Source: CAD feature listing. Evaluate the final solid. Frame: model axes, mm. Round coordinates to 2 decimals unless told otherwise and drop trailing zeros. Loops run counter-clockwise (first coordinate to the right, second up) from the corner with the lowest first, then second, coordinate; pieces in that order, holes last.
Item 1: Ray query, L1, parallel to Z at x = 95, y = 1.05; L2, parallel to X at y = 1.25, z = 52; L3, parallel to X at y = 4.15, z = -26 (3 decimals). Return the intervals inside material, ascending.
Item 2: Section query C-C on x = -34.5. Return loops of the section in (y, z).
Item 3: First-contact query: P1, Ø2.5, axis at x = -94.5, z = -52, coming from the +Y side; P2, Ø1.6, axis at y = 4, z = 14, coming from the +X side; P3, Ø0.6, axis at x = 50, y = 4.5, coming from the -Z side. Flat tips, straight axial feed; report the tip coordinate or a pass-through.
Item 4: Section query D-D on x = -80. Return loops of the section in (y, z).
Item 5: Section query B-B on y = 3.8. Return loops of the section in (x, z) (3 decimals), then the cut area to 3 significant figures.
Item 6: Section query A-A on z = -26. Return loops of the section in (x, y) (3 decimals).
```python
from build123d import *

# Parameters (mm, degrees)
SKETCH1_W           = 195
SKETCH1_H           = 110
BOSS_EXTRUDE1_DEPTH = 3
BOSS_EXTRUDE2_DEPTH = 2
SKETCH4_R           = 1.5
CUT_EXTRUDE2_DEPTH  = 112.983257677
FILLET1_R           = 3
SKETCH5_R           = 1.5
CUT_EXTRUDE3_DEPTH  = 113.054674155
SKETCH6_R           = 10.35
CUT_EXTRUDE4_DEPTH  = 113.054674155
SKETCH7_R           = 11.4
CUT_EXTRUDE5_DEPTH  = 2


with BuildPart() as part:
    # Sketch1 → Boss-Extrude1 (new body)
    with BuildSketch(Plane(origin=(0, 0, 0), x_dir=(1, 0, 0), z_dir=(0, 1, 0))):
        Rectangle(SKETCH1_W, SKETCH1_H)
    extrude(amount=BOSS_EXTRUDE1_DEPTH)

    # Sketch2 → Boss-Extrude2 (add)
    with BuildSketch(Plane(origin=(0, 3, 0), x_dir=(1, 0, 0), z_dir=(0, 1, 0))):
        with BuildLine():
            Line((-94.5, 0), (-94.5, 49))
            ThreePointArc((-94.5, 49), (-92.378679656, 49.878679656), (-91.5, 52))
            Line((-91.5, 52), (-13, 52))
            ThreePointArc((-13, 52), (-10.878679656, 51.121320344), (-10, 49))
            Line((-10, 49), (-10, -49))
            ThreePointArc((-10, -49), (-10.878679656, -51.121320344), (-13, -52))
            Line((-13, -52), (-91.5, -52))
            ThreePointArc((-91.5, -52), (-92.378679656, -49.878679656), (-94.5, -49))
            Line((-94.5, -49), (-94.5, 0))
        make_face()
        with BuildLine():
            Line((-7, 0), (-7, 49))
            ThreePointArc((-7, 49), (-6.121320344, 51.121320344), (-4, 52))
            Line((-4, 52), (92, 52))
            ThreePointArc((92, 52), (92.878679656, 49.878679656), (95, 49))
            Line((95, 49), (95, -49))
            ThreePointArc((95, -49), (92.878679656, -49.878679656), (92, -52))
            Line((92, -52), (-4, -52))
            ThreePointArc((-4, -52), (-6.121320344, -51.121320344), (-7, -49))
            Line((-7, -49), (-7, 0))
        make_face()
    extrude(amount=BOSS_EXTRUDE2_DEPTH)

    # Sketch4 → Cut-Extrude2 (cut, through all)
    with BuildSketch(Plane(origin=(0, 3, 0), x_dir=(1, 0, 0), z_dir=(0, 1, 0))):
        with Locations(Location((-94.5, 52, 0), (0, 0, 270))):
            Circle(SKETCH4_R)
        with Locations(Location((95, 52, 0), (0, 0, 270))):
            Circle(SKETCH4_R)
        with Locations(Location((95, -52, 0), (0, 0, 270))):
            Circle(SKETCH4_R)
        with Locations(Location((-94.5, -52, 0), (0, 0, 270))):
            Circle(SKETCH4_R)
    extrude(amount=-CUT_EXTRUDE2_DEPTH, mode=Mode.SUBTRACT)

    # Fillet1
    fillet1_edges = [part.edges().sort_by_distance(p)[0] for p in [
        (97.5, 1.5, 55),
        (-97.5, 1.5, 55),
        (-97.5, 1.5, -55),
        (97.5, 1.5, -55),
    ]]
    fillet(fillet1_edges, radius=FILLET1_R)

    # Sketch5 → Cut-Extrude3 (cut, through all)
    with BuildSketch(Plane(origin=(0, 5, 0), x_dir=(1, 0, 0), z_dir=(0, 1, 0))):
        with Locations(Location((-13, -49, 0), (0, 0, 270))):
            Circle(SKETCH5_R)
        with Locations(Location((-4, -49, 0), (0, 0, 270))):
            Circle(SKETCH5_R)
    extrude(amount=-CUT_EXTRUDE3_DEPTH, mode=Mode.SUBTRACT)

    # Sketch6 → Cut-Extrude4 (cut, through all)
    with BuildSketch(Plane(origin=(0, 5, 0), x_dir=(1, 0, 0), z_dir=(0, 1, 0))):
        with Locations(Location((-73.375, 26, 0), (0, 0, 270))):
            Circle(SKETCH6_R)
    extrude(amount=-CUT_EXTRUDE4_DEPTH, mode=Mode.SUBTRACT)

    # Sketch7 → Cut-Extrude5 (cut)
    with BuildSketch(Plane.XZ):
        with Locations(Location((-73.375, -26, 0), (0, 0, 270))):
            Circle(SKETCH7_R)
    extrude(amount=-CUT_EXTRUDE5_DEPTH, mode=Mode.SUBTRACT)


solid = part.part
```
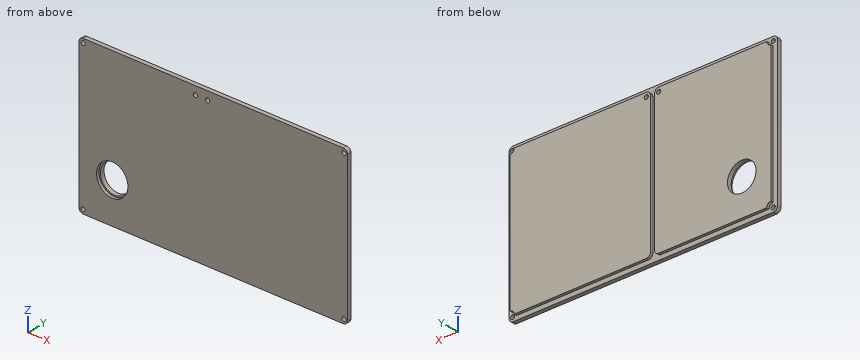
Data:
1. L1: z = -54.96 to -53.5, -50.5 to 50.5, 53.5 to 54.96
1. L2: x = -97.5 to -96, -93 to 93.5, 96.5 to 97.5
1. L3: x = -94.5 to -83.725, -63.025 to -10, -7 to 95
2. outline: (0, -55) - (3, -55) - (3, -52) - (5, -52) - (5, 52) - (3, 52) - (3, 55) - (0, 55) - close
3. P1: passes through
3. P2: stops at x = 95
3. P3: stops at z = -52
4. outline: (0, -55) - (3, -55) - (3, -52) - (5, -52) - (5, -33.95) - (2, -33.95) - (2, -35.28) - (0, -35.28) - close; (0, -16.72) - (2, -16.72) - (2, -18.05) - (5, -18.05) - (5, 52) - (3, 52) - (3, 55) - (0, 55) - close
5. outline: (-94.5, -49) arc R3 cw to (-91.5, -52) - (-13, -52) arc R3 ccw to (-10, -49) - (-10, 49) arc R3 ccw to (-13, 52) - (-91.5, 52) arc R3 cw to (-94.5, 49) - close; (-7, -49) arc R3 ccw to (-4, -52) - (92, -52) arc R3 cw to (95, -49) - (95, 49) arc R3 cw to (92, 52) - (-4, 52) arc R3 ccw to (-7, 49) - close; hole circle Ø20.7 at (-73.375, -26); hole circle Ø3 at (-13, 49); hole circle Ø3 at (-4, 49)
5. area: 19,000 mm2
6. outline: (-97.5, 0) - (-84.775, 0) - (-84.775, 2) - (-83.725, 2) - (-83.725, 5) - (-94.5, 5) - (-94.5, 3) - (-97.5, 3) - close; (-63.025, 2) - (-61.975, 2) - (-61.975, 0) - (97.5, 0) - (97.5, 3) - (95, 3) - (95, 5) - (-7, 5) - (-7, 3) - (-10, 3) - (-10, 5) - (-63.025, 5) - close
